```python
from build123d import *

# Parameters (mm, degrees)
SKETCH1_R                      = 4.5
BOSS_EXTRUDE1_DEPTH            = 32
SKETCH1_4_R                    = 4.5
BOSS_EXTRUDE2_DEPTH            = 9
M3_CLEARANCE_HOLE1_D           = 3.6
M3_CLEARANCE_HOLE1_CSINK_D     = 3.65
M3_CLEARANCE_HOLE1_CSINK_ANGLE = 90
FILLET1_R                      = 1


with BuildPart() as part:
    # Sketch1 → Boss-Extrude1 (new body)
    with BuildSketch(Plane(origin=(0, 0, 0), x_dir=(1, 0, 0), z_dir=(0, 1, 0))):
        with Locations(Location((0, 0, 0), (0, 0, 270))):
            Circle(SKETCH1_R)
        with BuildLine():
            Line((-2.4, -0.885640646), (-2.4, 0.885640646))
            ThreePointArc((-2.4, 0.885640646), (-2.833012702, 1.635640646), (-1.966987298, 1.635640646))
            Line((-1.966987298, 1.635640646), (-0.433012702, 2.521281292))
            ThreePointArc((-0.433012702, 2.521281292), (-0.129409523, 3.254244205), (0.5, 2.771281292))
            ThreePointArc((0.5, 2.771281292), (0.482962913, 2.64187177), (0.433012702, 2.521281292))
            Line((0.433012702, 2.521281292), (1.966987298, 1.635640646))
            ThreePointArc((1.966987298, 1.635640646), (2.529409523, 1.868603559), (2.9, 1.385640646))
            ThreePointArc((2.9, 1.385640646), (2.753553391, 1.032087255), (2.4, 0.885640646))
            Line((2.4, 0.885640646), (2.4, -0.885640646))
            ThreePointArc((2.4, -0.885640646), (2.753553391, -1.032087255), (2.9, -1.385640646))
            ThreePointArc((2.9, -1.385640646), (2.529409523, -1.868603559), (1.966987298, -1.635640646))
            Line((1.966987298, -1.635640646), (0.433012702, -2.521281292))
            ThreePointArc((0.433012702, -2.521281292), (0.482962913, -2.64187177), (0.5, -2.771281292))
            ThreePointArc((0.5, -2.771281292), (-0.129409523, -3.254244205), (-0.433012702, -2.521281292))
            Line((-0.433012702, -2.521281292), (-1.966987298, -1.635640646))
            ThreePointArc((-1.966987298, -1.635640646), (-2.833012702, -1.635640646), (-2.4, -0.885640646))
        make_face(mode=Mode.SUBTRACT)
    extrude(amount=BOSS_EXTRUDE1_DEPTH)

    # Sketch1_4 → Boss-Extrude2 (add)
    with BuildSketch(Plane(origin=(0, 0, 0), x_dir=(1, 0, 0), z_dir=(0, 1, 0))):
        with Locations(Location((0, 0, 0), (0, 0, 270))):
            Circle(SKETCH1_4_R)
    extrude(amount=BOSS_EXTRUDE2_DEPTH)

    # M3 Clearance Hole1 (through all)
    with Locations(Plane(origin=(0, 0, 0), x_dir=(-1, 0, 0), z_dir=(0, -1, 0))):
        with Locations((0, 0)):
            CounterSinkHole(M3_CLEARANCE_HOLE1_D / 2, M3_CLEARANCE_HOLE1_CSINK_D / 2, counter_sink_angle=M3_CLEARANCE_HOLE1_CSINK_ANGLE)

    # Fillet1
    fillet1_edges = [part.edges().sort_by_distance(p)[0] for p in [
        (-2.4, 20.5, -0.885640646),
        (-2.4, 20.5, 0.885640646),
        (-1.966987298, 20.5, 1.635640646),
        (-0.433012702, 20.5, 2.521281292),
        (0.433012702, 20.5, 2.521281292),
        (1.966987298, 20.5, 1.635640646),
        (2.4, 20.5, 0.885640646),
        (2.4, 20.5, -0.885640646),
        (1.966987298, 20.5, -1.635640646),
        (0.433012702, 20.5, -2.521281292),
        (-0.433012702, 20.5, -2.521281292),
        (-1.966987298, 20.5, -1.635640646),
    ]]
    fillet(fillet1_edges, radius=FILLET1_R)


solid = part.part
```
Read the model definition and answer for the solid it produces. Units are mm, in the model's axes. A direction names the side the tool comes from. Coordinates: 2 decimals unless noted, no trailing zeros. Loops run counter-clockwise (first coordinate to the right, second up) from the corner with the lowest first, then second, coordinate; pieces in that order, holes last.
(1) A tool of negligible diameter and unlimited length cuts with its end or side. For faces 5 (the face through (1.717, 4.575, -0.541)), 6 (the face through (0.01, 20.34, 3.27)), from which of +Z, -Z, +X, -X, +Y, -Y can it reach the whole face along a straight path? Write none if from no direction.
Solution:
face 5: +Y, -Y
face 6: +Y
(2) The part is cut by section B-B (y = 8). Determine the outline of the cut face in (x, z), and give its area (3 significant figures).
Solution:
outline: circle Ø9 at (0, 0); hole circle Ø3.6 at (0, 0)
area: 53.4 mm2
(3) Consider line 1 along Z through (x, y) = (-2.75, 22); line 2 along Y through (x, z) = (0.75, -2); line 3 along X through (y, z) = (24, 1.5). Determine where each line is inside the solid, lowest interval first.
Solution:
line 1: z = -3.56 to -1.74, -1.03 to 1.03, 1.74 to 3.56
line 2: y = 0 to 9
line 3: x = -4.24 to -2.89, 2.89 to 4.24
(4) The mould has two halves that part along Z. Classify faces 1 (the face through (1.352, 15.776, 4.292)), 2 (the face through (-2, 9, 1)), 3 (the face through (-2, 32, 2)), 4 (the face through (1.823, 20.661, -1.817)): released by +Z, released by -Z, zero draft, split by the parting line, or undercut.
Solution:
face 1: split by the parting line
face 2: undercut
face 3: zero draft
face 4: undercut
(5) The part is cut by section C-C (x = 3.5). Determine the outline of the cut face in (y, z), and give its area (3 significant figures).
Solution:
outline: (0, -2.83) - (32, -2.83) - (32, 2.83) - (0, 2.83) - close
area: 181 mm2
(6) The part is cut by section A-A (x = 0). Determine the outline of the cut face in (y, z) (3 decimals), and give its area (3 significant figures).
Solution:
outline: (0, -4.5) - (32, -4.5) - (32, -3.271) - (9, -3.271) - (9, -1.8) - (0.025, -1.8) - (0, -1.825) - close; (0, 1.825) - (0.025, 1.8) - (9, 1.8) - (9, 3.271) - (32, 3.271) - (32, 4.5) - (0, 4.5) - close
area: 105 mm2
(7) Flat-ended cylindrical pins translate along their axes: pin 1 Ø5 at (x, y) = (-2.5, 20.5) entering from -Z; pin 2 Ø1.7 at (x, z) = (0, 1) entering from +Y; pin 3 Ø1 at (y, z) = (11, 2.5) entering from -X. Find the tip coordinate at first contact, or state that the pin passes through.
Solution:
pin 1: stops at z = -4.5
pin 2: stops at y = 9
pin 3: stops at x = -4.03
